Print and shaded views of the part. All mm, measured from the part's lowest x, y and z. A direction names the side the tool comes from. Round coordinates to 2 decimals unless told otherwise and drop trailing zeros. Loops run counter-clockwise (first coordinate to the right, second up) from the corner with the lowest first, then second, coordinate; pieces in that order, holes last. Notation, with made-up numbers: (21.5, 66.5) - (54.5, 66.5) arc R24 ccw to (54.5, 82.5) - close; hole circle Ø2 at (12, 22.25). An arc over 180 degrees is marked (long way). Answer as a JSON object with one key per item and string values.
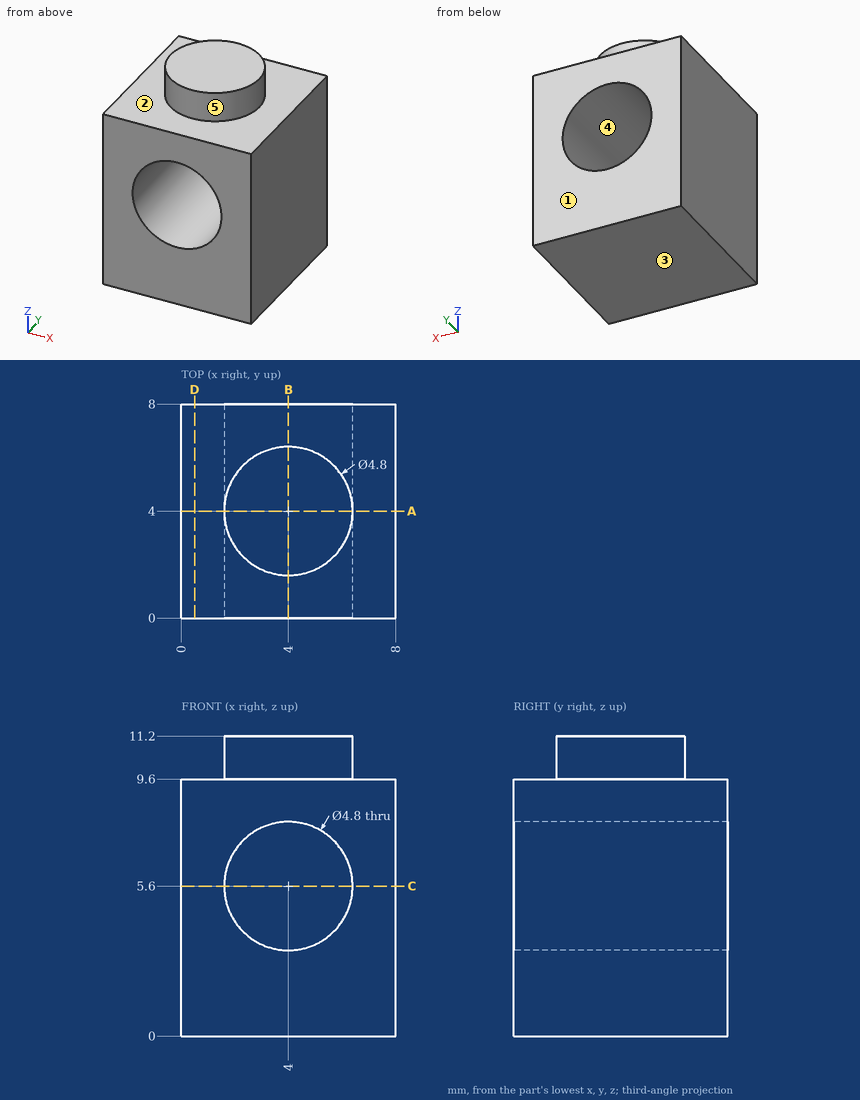
1) Slice it at B-B on x = 4. List the corners of the cut face in (y, z).
Values follow:
{"outline": "(0, 0) - (8, 0) - (8, 3.2) - (0, 3.2) - close; (0, 8) - (8, 8) - (8, 9.6) - (6.4, 9.6) - (6.4, 11.2) - (1.6, 11.2) - (1.6, 9.6) - (0, 9.6) - close"}
2) Slice it at D-D on x = 0.5. List the corners of the cut face in (y, z).
Values follow:
{"outline": "(0, 0) - (8, 0) - (8, 9.6) - (0, 9.6) - close"}
3) Slice it at C-C on z = 5.6. List the corners of the cut face in (x, y), then the cut area to 3 significant figures.
Values follow:
{"outline": "(0, 0) - (1.6, 0) - (1.6, 8) - (0, 8) - close; (6.4, 0) - (8, 0) - (8, 8) - (6.4, 8) - close", "area": "25.6 mm²"}
4) Tool access for the marked faces 1 and 2: list every direction of +Z, -Z, +X, -X, +Y, -Y with a clear straight run to the whole face (end or side of a thin tool).
Values follow:
{"face 1": "+Z, -Z, +X, -X, +Y", "face 2": "+Z"}
5) Two-plate mould, pull along X, no slides. Class the marked faces 3, 4 and 5: pulls with the +X half, pulls with the -X half, needs draft (parallel to the pull), parting line crosses it, or undercut.
Values follow:
{"face 3": "needs draft", "face 4": "undercut", "face 5": "parting line crosses it"}
6) Probe probe 1 along X at (y, z) = (6.25, 5.5); probe 2 along Z at (x, y) = (4, 5.75); probe 3 along Z at (x, y) = (0.5, 2.75). List the from-to ranges inside material, lowest first.
Values follow:
{"probe 1": "0 to 1.6, 6.4 to 8", "probe 2": "0 to 3.2, 8 to 11.2", "probe 3": "0 to 9.6"}
7) Slice it at A-A on y = 4. List the corners of the cut face in (x, z), then the cut area to 3 significant figures.
Values follow:
{"outline": "(0, 0) - (8, 0) - (8, 9.6) - (6.4, 9.6) - (6.4, 11.2) - (1.6, 11.2) - (1.6, 9.6) - (0, 9.6) - close; hole circle Ø4.8 at (4, 5.6)", "area": "66.4 mm²"}
